```python
from build123d import *

# Parameters (mm, degrees)
AUFSATZ_LINEAR_AUSTRAGEN1_DEPTH = 2
AUFSATZ_LINEAR_AUSTRAGEN2_DEPTH = 2


with BuildPart() as part:
    # Skizze1 → Aufsatz-Linear austragen1 (new body)
    with BuildSketch(Plane.XY.offset(14.58852)):
        Polygon((-22.149859894, 27.765281808), (-55.023633975, 46.732102334), (-65.619428736, 28.349034811), (-33.1799992, 9.582671858), (-33.1799992, -9.82193495), (-65.441180026, -28.458395245), (-54.832668225, -46.841377939), (-21.94526311, -27.869445957), (-11.635211495, -33.81000048), (-10.63000112, -33.81000048), (-10.63000112, -70.99999976), (10.588764643, -70.99999976), (10.608764603, -33.81000048), (11.636228403, -33.81000048), (21.961456264, -27.849347945), (54.791716349, -46.801638497), (65.402118422, -28.428154068), (36.372671479, -11.66999904), (37.79000014, -11.66999904), (37.79000014, 11.41999954), (35.875483821, 11.41999954), (65.431940836, 28.488460753), (54.822266278, 46.860690996), (21.946878227, 27.90320319), (11.612735063, 33.83000044), (10.5900012, 33.83000044), (10.5900012, 70.94999986), (-10.65000108, 70.94999986), (-10.65000108, 33.83000044), (-11.635793215, 33.83000044), align=None)
    extrude(amount=AUFSATZ_LINEAR_AUSTRAGEN1_DEPTH)

    # Skizze2 → Aufsatz-Linear austragen2 (add)
    with BuildSketch(Plane(origin=(0, 0, 14.58852), x_dir=(-1, 0, 0), z_dir=(0, 0, -1))):
        Polygon((29.5799992, 9.810611271), (29.5799992, -10.052032223), (62.709719012, -29.19022531), (54.099914325, -44.109744044), (21.94585632, -25.560861902), (11.100245691, -31.81000048), (8.63000112, -31.81000048), (8.63000112, -68.99999976), (-8.58983991, -68.99999976), (-8.60983987, -31.81000048), (-11.100378331, -31.81000048), (-21.96144846, -25.540011472), (-54.059788028, -44.0697781), (-62.669841481, -29.160193905), (-28.907796867, -9.66999904), (-11.412909471, -9.66999904), (-11.412909471, 9.41999954), (-28.412909471, 9.41999954), (-62.699818266, 29.220233802), (-54.089861915, 44.129654408), (-21.949592186, 25.596070242), (-11.079922713, 31.83000044), (-8.5900012, 31.83000044), (-8.5900012, 68.94999986), (8.65000108, 68.94999986), (8.65000108, 31.83000044), (11.100321567, 31.83000044), (22.149980751, 25.45634161), (54.290039962, 43.999838722), (62.88949027, 29.080308923), align=None)
    extrude(amount=AUFSATZ_LINEAR_AUSTRAGEN2_DEPTH)


solid = part.part
```
The model under review builds one solid part; all positions refer to its coordinate system, in mm. A direction names the side the tool comes from. Round coordinates to 2 decimals unless told otherwise and drop trailing zeros. Write each loop counter-clockwise with the first axis right and the second up, starting at its lowest first coordinate (ties: lowest second). Pieces come first, ordered by that corner, then holes. Notation, with made-up numbers: (56, 71.5) - (63, 71.5) arc R4 ccw to (63, 75.5) - close; hole circle Ø9 at (38, -23.75). An arc over 180 degrees is marked (long way). One line per question, with ' | ' between items.
Item 1: For P1, Ø1.6, axis at x = -1.5, z = 13.5, coming from the +Y side; P2, Ø2, axis at y = 54.5, z = 15.5, coming from the +X side; P3, Ø0.8, axis at x = -11.5, z = 15.5, coming from the +Y side, all flat-tipped, find the tip position at first contact; note any pin that passes through.
Resolved:
P1: stops at y = 68.95 | P2: stops at x = 10.59 | P3: stops at y = 33.83
Item 2: The part is to be moulded in two halves that separate along Y. For faces 5 (the face through (58.455, 36.571, 13.603)), 6 (the face through (46.025, -19.552, 13.603)), 7 (the face through (38.147, -37.193, 15.575)), say which applies: pulls with the +Y half, pulls with the -Y half, needs draft (parallel to the pull), parting line crosses it, or undercut.
Resolved:
face 5: pulls with the +Y half | face 6: undercut | face 7: pulls with the -Y half
Item 3: Add section C-C, the plane y = 22. Give the boundary of the cut face in (x, z), then the cut area to 3 significant figures.
Resolved:
outline: (-54.64, 14.59) - (-50.65, 14.59) - (-50.65, 12.59) - (50.2, 12.59) - (50.2, 14.59) - (54.2, 14.59) - (54.2, 16.59) - (-54.64, 16.59) - close | area: 419 mm2
Item 4: Add section A-A, the plane y = -2. Give the boundary of the cut face in (x, z).
Resolved:
outline: (-33.18, 14.59) - (-29.58, 14.59) - (-29.58, 12.59) - (11.41, 12.59) - (11.41, 14.59) - (37.79, 14.59) - (37.79, 16.59) - (-33.18, 16.59) - close
Item 5: To check wall thickness, follow probe 1 along X at (y, z) = (-38, 16.45) (3 decimals); probe 2 along X at (y, z) = (-40.5, 15.2); probe 3 along Y at (x, z) = (-58, 13.6). State the ranges of each line that lie inside material, in increasing order.
Resolved:
probe 1: x = -59.935 to -39.506, -10.63 to 10.607, 39.545 to 59.875 | probe 2: x = -58.49 to -43.84, -10.63 to 10.61, 43.88 to 58.43 | probe 3: y = -37.35 to -26.47, 26.25 to 37.56
Item 6: For faces 1 (the face through (-16.82, 30.84, 15.57)), 2 (the face through (16.59, 28.67, 13.6)), 3 (the face through (58.305, -36.719, 13.603)), 4 (the face through (37.786, -34.675, 13.603)), list the 3-axis set-ups (+Z, -Z, +X, -X, +Y, -Y) from which the entire face can be reached by the end or side of a thin tool; tool diameter is ignored.
Resolved:
face 1: +Z, -Z, +Y | face 2: -Z, +Y | face 3: -Z, +X, -Y | face 4: -Z, -Y
